```python
from build123d import *

# Parameters (mm, degrees)
SKETCH1_W                      = 60
SKETCH1_H                      = 388.5
BASE_FLANGE1_DEPTH             = 4
EDGE_FLANGE1_STRIP_W           = 18
EDGE_FLANGE1_STRIP_H           = 4
EDGE_FLANGE1_STRIP_CUT_DEPTH   = 388.5
EDGE_FLANGE1_DEPTH             = 388.5
EDGE_FLANGE2_STRIP_W           = 18
EDGE_FLANGE2_STRIP_H           = 4
EDGE_FLANGE2_STRIP_CUT_DEPTH   = 55
EDGE_FLANGE2_STRIP_2_W         = 18
EDGE_FLANGE2_STRIP_2_H         = 4
EDGE_FLANGE2_STRIP_CUT_2_DEPTH = 55
EDGE_FLANGE2_STRIP_3_W         = 18
EDGE_FLANGE2_STRIP_3_H         = 4
EDGE_FLANGE2_STRIP_CUT_3_DEPTH = 55
EDGE_FLANGE2_STRIP_4_W         = 18
EDGE_FLANGE2_STRIP_4_H         = 4
EDGE_FLANGE2_STRIP_CUT_4_DEPTH = 55
EDGE_FLANGE2_DEPTH             = 55
EDGE_FLANGE2_BEND_DEPTH        = 55
EDGE_FLANGE2_BEND_2_DEPTH      = 55
EDGE_FLANGE2_BEND_3_DEPTH      = 55
SKETCH18_R                     = 4.6
EXTRUDE1_DEPTH                 = 399.607890037
SKETCH19_R                     = 4.6
EXTRUDE2_DEPTH                 = 4
SKETCH20_R                     = 4.6
EXTRUDE3_DEPTH                 = 4


# Sheet-metal steps are written as plain solids
with BuildPart() as part:
    # Sketch1 → Base-Flange1 (new body)
    with BuildSketch(Plane(origin=(0, 0, 0), x_dir=(1, 0, 0), z_dir=(0, 1, 0))):
        Rectangle(SKETCH1_W, SKETCH1_H)
    extrude(amount=BASE_FLANGE1_DEPTH)

    # Edge-Flange1 strip (across the edge) → Edge-Flange1 strip cut (cut)
    with BuildSketch(Plane(origin=(-30, 4, -194.25), x_dir=(1, 0, 0), z_dir=(0, 0, 1))):
        with Locations((-4, -2)):
            Rectangle(EDGE_FLANGE1_STRIP_W, EDGE_FLANGE1_STRIP_H)
    extrude(amount=EDGE_FLANGE1_STRIP_CUT_DEPTH, mode=Mode.SUBTRACT)

    # Edge-Flange1 section (across the edge) → Edge-Flange1 (add)
    with BuildSketch(Plane(origin=(-30, 4, -194.25), x_dir=(1, 0, 0), z_dir=(0, 0, 1))):
        with BuildLine():
            Line((0, 1), (0, 56))
            Line((0, 56), (4, 56))
            Line((4, 56), (4, 1))
            ThreePointArc((4, 1), (4.292893219, 0.292893219), (5, 0))
            Line((5, 0), (5, -4))
            ThreePointArc((5, -4), (1.464466094, -2.535533906), (0, 1))
        make_face()
    extrude(amount=EDGE_FLANGE1_DEPTH)

    # Edge-Flange2 strip (across the edge) → Edge-Flange2 strip cut (cut)
    with BuildSketch(Plane(origin=(-30, 5, 194.25), x_dir=(0, 0, -1), z_dir=(0, 1, 0))):
        with Locations((-4, -2)):
            Rectangle(EDGE_FLANGE2_STRIP_W, EDGE_FLANGE2_STRIP_H)
    extrude(amount=EDGE_FLANGE2_STRIP_CUT_DEPTH, mode=Mode.SUBTRACT)

    # Edge-Flange2 strip 2 (across the edge) → Edge-Flange2 strip cut 2 (cut)
    with BuildSketch(Plane(origin=(30, 0, 194.25), x_dir=(0, 0, -1), z_dir=(-1, 0, 0))):
        with Locations((-4, -2)):
            Rectangle(EDGE_FLANGE2_STRIP_2_W, EDGE_FLANGE2_STRIP_2_H)
    extrude(amount=EDGE_FLANGE2_STRIP_CUT_2_DEPTH, mode=Mode.SUBTRACT)

    # Edge-Flange2 strip 3 (across the edge) → Edge-Flange2 strip cut 3 (cut)
    with BuildSketch(Plane(origin=(-30, 60, -194.25), x_dir=(0, 0, 1), z_dir=(0, -1, 0))):
        with Locations((-4, -2)):
            Rectangle(EDGE_FLANGE2_STRIP_3_W, EDGE_FLANGE2_STRIP_3_H)
    extrude(amount=EDGE_FLANGE2_STRIP_CUT_3_DEPTH, mode=Mode.SUBTRACT)

    # Edge-Flange2 strip 4 (across the edge) → Edge-Flange2 strip cut 4 (cut)
    with BuildSketch(Plane(origin=(-25, 0, -194.25), x_dir=(0, 0, 1), z_dir=(1, 0, 0))):
        with Locations((-4, -2)):
            Rectangle(EDGE_FLANGE2_STRIP_4_W, EDGE_FLANGE2_STRIP_4_H)
    extrude(amount=EDGE_FLANGE2_STRIP_CUT_4_DEPTH, mode=Mode.SUBTRACT)

    # Edge-Flange2 section (across the edge) → Edge-Flange2 (add)
    with BuildSketch(Plane(origin=(-30, 5, 194.25), x_dir=(0, 0, -1), z_dir=(0, 1, 0))):
        with BuildLine():
            Line((0, 1), (0, 36))
            Line((0, 36), (4, 36))
            Line((4, 36), (4, 1))
            ThreePointArc((4, 1), (4.292893219, 0.292893219), (5, 0))
            Line((5, 0), (5, -4))
            ThreePointArc((5, -4), (1.464466094, -2.535533906), (0, 1))
        make_face()
    extrude(amount=EDGE_FLANGE2_DEPTH)

    # Edge-Flange2 section 2 (across the edge) → Edge-Flange2 bend (add)
    with BuildSketch(Plane(origin=(30, 0, 194.25), x_dir=(0, 0, -1), z_dir=(-1, 0, 0))):
        with BuildLine():
            Line((0, 1), (0, 36))
            Line((0, 36), (4, 36))
            Line((4, 36), (4, 1))
            ThreePointArc((4, 1), (4.292893219, 0.292893219), (5, 0))
            Line((5, 0), (5, -4))
            ThreePointArc((5, -4), (1.464466094, -2.535533906), (0, 1))
        make_face()
    extrude(amount=EDGE_FLANGE2_BEND_DEPTH)

    # Edge-Flange2 section 3 (across the edge) → Edge-Flange2 bend 2 (add)
    with BuildSketch(Plane(origin=(-30, 60, -194.25), x_dir=(0, 0, 1), z_dir=(0, -1, 0))):
        with BuildLine():
            Line((0, 1), (0, 36))
            Line((0, 36), (4, 36))
            Line((4, 36), (4, 1))
            ThreePointArc((4, 1), (4.292893219, 0.292893219), (5, 0))
            Line((5, 0), (5, -4))
            ThreePointArc((5, -4), (1.464466094, -2.535533906), (0, 1))
        make_face()
    extrude(amount=EDGE_FLANGE2_BEND_2_DEPTH)

    # Edge-Flange2 section 4 (across the edge) → Edge-Flange2 bend 3 (add)
    with BuildSketch(Plane(origin=(-25, 0, -194.25), x_dir=(0, 0, 1), z_dir=(1, 0, 0))):
        with BuildLine():
            Line((0, 1), (0, 36))
            Line((0, 36), (4, 36))
            Line((4, 36), (4, 1))
            ThreePointArc((4, 1), (4.292893219, 0.292893219), (5, 0))
            Line((5, 0), (5, -4))
            ThreePointArc((5, -4), (1.464466094, -2.535533906), (0, 1))
        make_face()
    extrude(amount=EDGE_FLANGE2_BEND_3_DEPTH)

    # Sketch18 → Extrude1 (cut, through all)
    with BuildSketch(Plane.XY.offset(194.25)):
        with Locations((-46, 47.5)):
            Circle(SKETCH18_R)
        with Locations((-46, 17.5)):
            Circle(SKETCH18_R)
        with Locations((-12.5, -16)):
            Circle(SKETCH18_R)
        with Locations((17.5, -16)):
            Circle(SKETCH18_R)
    extrude(amount=-EXTRUDE1_DEPTH, mode=Mode.SUBTRACT)

    # Sketch19 → Extrude2 (cut)
    with BuildSketch(Plane(origin=(-26, 0, 0), x_dir=(0, 0, -1), z_dir=(1, 0, 0))):
        with Locations(Location((-114.25, 35, 0), (0, 0, 90))):
            Circle(SKETCH19_R)
        with Locations(Location((114.25, 35, 0), (0, 0, 90))):
            Circle(SKETCH19_R)
    extrude(amount=-EXTRUDE2_DEPTH, mode=Mode.SUBTRACT)

    # Sketch20 → Extrude3 (cut)
    with BuildSketch(Plane(origin=(0, 4, 0), x_dir=(1, 0, 0), z_dir=(0, 1, 0))):
        with Locations(Location((5, 114.25, 0), (0, 0, 270))):
            Circle(SKETCH20_R)
        with Locations(Location((5, -114.25, 0), (0, 0, 270))):
            Circle(SKETCH20_R)
    extrude(amount=-EXTRUDE3_DEPTH, mode=Mode.SUBTRACT)


solid = part.part
```
Input: part model. Units: mm. Frame: model coordinates. A direction names the side the tool comes from. Give positions to 0.01 mm unless a question says otherwise; leave off trailing zeros. Order: outer loops, then holes, each group sorted by start corner. A loop starts at its lowest first (then second) coordinate and runs counter-clockwise, first axis right, second up. Notation, with made-up numbers: M 67,36.25 L 120,36.25 A11 ccw 120,48.25 Z; hole C -22.75,14.5 d2. An arc over 180 degrees is marked long. Return JSON: item names as keys, results as strings.
1) Section query A-A on z = -114.25. Output: boundary loops of the cut face in (x, y).
Taken from the geometry:
{"outline": "M -30,5 A5 ccw -25,0 L 0.4,0 L 0.4,4 L -25,4 A1 cw -26,5 L -26,30.4 L -30,30.4 Z; M -30,39.6 L -26,39.6 L -26,60 L -30,60 Z; M 9.6,0 L 30,0 L 30,4 L 9.6,4 Z"}
2) Access query for faces 1 (the face through (-43.53, 21.38, 192.28)), 2 (the face through (2, -19, -190.25)), 3 (the face through (-26, 33, -3)), 4 (the face through (-30, 32, -3)). Directions: +Z, -Z, +X, -X, +Y, -Y. A direction counts if a zero-diameter tool reaches every point of the face in a straight line with its end or side. Return the directions, or none.
Taken from the geometry:
{"face 1": "+Z, -Z", "face 2": "+X, -X, -Y", "face 3": "+Z, -Z, +X, +Y", "face 4": "-X, +Y, -Y"}
3) Section query C-C on y = 47.5. Output: boundary loops of the cut face in (x, z).
Taken from the geometry:
{"outline": "M -66,-194.25 L -50.6,-194.25 L -50.6,-190.25 L -66,-190.25 Z; M -66,190.25 L -50.6,190.25 L -50.6,194.25 L -66,194.25 Z; M -41.4,-194.25 L -31,-194.25 A5 ccw -26,-189.25 L -26,189.25 A5 ccw -31,194.25 L -41.4,194.25 L -41.4,190.25 L -31,190.25 A1 cw -30,189.25 L -30,-189.25 A1 cw -31,-190.25 L -41.4,-190.25 Z"}
4) Section query D-D on x = -12.5. Output: boundary loops of the cut face in (y, z), and give its area (3 significant figures).
Taken from the geometry:
{"outline": "M -36,-194.25 L -20.6,-194.25 L -20.6,-190.25 L -36,-190.25 Z; M -36,190.25 L -20.6,190.25 L -20.6,194.25 L -36,194.25 Z; M -11.4,-194.25 L -1,-194.25 A5 ccw 4,-189.25 L 4,189.25 A5 ccw -1,194.25 L -11.4,194.25 L -11.4,190.25 L -1,190.25 A1 cw 0,189.25 L 0,-189.25 A1 cw -1,-190.25 L -11.4,-190.25 Z", "area": "1,760 mm2"}
5) Mould query, pull axis Y, two halves, no side actions, for faces 5 (the face through (3, -18, 194.25)), 6 (the face through (-28, 60, 1)), 7 (the face through (-10.03, -12.12, -192.22)). Classes: released by +Y, released by -Y, zero draft, split by the parting line, or undercut.
Taken from the geometry:
{"face 5": "zero draft", "face 6": "released by +Y", "face 7": "undercut"}
6) Section query B-B on x = -56.5. Output: boundary loops of the cut face in (y, z), and give its area (3 significant figures).
Taken from the geometry:
{"outline": "M 5,-194.25 L 60,-194.25 L 60,-190.25 L 5,-190.25 Z; M 5,190.25 L 60,190.25 L 60,194.25 L 5,194.25 Z", "area": "440 mm2"}
7) Contact query for flat-ended pins moving along their axis: pin 1 (5.5 mm diameter, centred on x = -51.5, z = -191, fed in from -Y); pin 2 (2 mm diameter, centred on y = 17, z = 89, fed in from -X). Output: stop coordinate, or through.
Taken from the geometry:
{"pin 1": "stops at y = 5", "pin 2": "stops at x = -30"}
8) Line query: L1, parallel to Y at x = -46, z = 192; L2, parallel to Z at x = -57, y = 43.5; L3, parallel to Y at x = 26, z = -129. Output: solid intervals per line, ascending. Write a range as [from, to].
Taken from the geometry:
{"L1": "y = [5, 12.9], [22.1, 42.9], [52.1, 60]", "L2": "z = [-194.25, -190.25], [190.25, 194.25]", "L3": "y = [0, 4]"}
